Autodesk Inventor part; units mm, degrees
ref_plane "YZ Plane" through (0, 0, 0) normal (1, 0, 0) x (0, 1, 0)
ref_plane "XZ Plane" through (0, 0, 0) normal (0, 1, 0) x (-1, 0, 0)
ref_plane "XY Plane" through (0, 0, 0) normal (0, 0, 1) x (1, 0, 0)
sketch "Sketch3" plane through (0, 0, 0) normal (0, 0, 1) x (1, 0, 0)
  circle A0 centre (0, 0) radius 10.4
  circle A1 centre (-7.9, 0) radius 0.975
  circle A2 centre (7.9, 0) radius 0.975
  circle A3 centre (-7.9, 0) radius 0.975
  circle A4 centre (7.9, 0) radius 0.975
  dimension "d0" = 20.8
extrude "Extrusion1" add sketch "Sketch3" along normal blind 2.4
sketch "Sketch4" plane through (0, 0, 0) normal (0, 0, -1) x (-1, 0, 0)
  circle A0 centre (0, 0) radius 4.35
  circle A1 centre (0, 0) radius 2.7
  dimension "d3" = 8.7
  dimension "d4" = 5.4
extrude "Extrusion2" add sketch "Sketch4" along normal blind 3 contours A0 | A1
sketch "Sketch5" plane through (0, 0, -3) normal (0, 0, -1) x (-1, 0, 0)
  circle A0 centre (0, 0) radius 2.75
  dimension "d7" = 5.5
extrude "Extrusion3" cut sketch "Sketch5" against normal blind 2.1
sketch "Sketch6" plane through (0, 0, 2.4) normal (0, 0, 1) x (1, 0, 0)
  circle A0 centre (0, 0) radius 2.85
  dimension "d10" = 5.7
extrude "Extrusion4" cut sketch "Sketch6" against normal blind 1
sketch "Sketch7" plane through (0, 0, 1.4) normal (0, 0, 1) x (1, 0, 0)
  circle A0 centre (0, 0) radius 4.35
  circle A1 centre (0, 0) radius 1.5
  dimension "d13" = 3
extrude "Extrusion5" cut sketch "Sketch7" against normal through all contours A1
properties part number "Circulo_Inferior"
The listing builds one solid part. Answer for the finished solid, in the listing's coordinates (mm). A direction names the side the tool comes from. Coordinates: 2 decimals unless noted, no trailing zeros. Order: outer loops, then holes, each group sorted by start corner. A loop starts at its lowest first (then second) coordinate and runs counter-clockwise, first axis right, second up. Notation, with made-up numbers: (46.25, 55) -> (102.25, 55) arc R18 ccw to (102.25, 89) -> close; hole circle Ø10 at (36.25, 55). An arc over 180 degrees is marked (long way). Answer in a Markdown table with one row per item. Add a question column.
Item 1: Find section B-B (x = 0). Write down the section's boundary in (y, z).
Item 2: Find section C-C (z = -0.3). Write down the section's boundary in (x, y), then the cut area to 3 significant figures.
Item 3: Find section A-A (y = 0). Write down the section's boundary in (x, z) (3 decimals), then the cut area to 3 significant figures.
Item 4: Find the intervals of material crossed by L1, parallel to Y at x = 0, z = 1.75; L2, parallel to Y at x = 0, z = -2.25; L3, parallel to Z at x = -6.5, y = -4.25, in increasing order. Write a range as from..to.
Item 5: Determine the mould class of faces 1 (the face through (1.2, -1.2, 1.4)), 2 (the face through (0.943, 4.247, -1.479)), 3 (the face through (2.2, -2.2, 2.4)) for opening direction X: +X half, -X half, draft (parallel to the pull), parting line (faces both ways), or undercut.
Item 6: Which of the six approach directions +Z, -Z, +X, -X, +Y, -Y give full straight-line access (tool end or side, diameter ignored) to faces 4 (the face through (4.5, 0.1, 0)), 5 (the face through (-2.262, -1.734, 1.907)), 6 (the face through (8.83, -0.29, 1.18))?
Item 7: Find section D-D (y = -4). Write down the section's boundary in (x, z), then the cut area to 3 significant figures.
Item 8: Each of these flat-tipped pins is pushed along its axis until it touches: P1, Ø6.5, axis at x = -0.5, y = -1, coming from the +Z side; P2, Ø1, axis at x = -3, z = -2, coming from the +Y side; P3, Ø5, axis at x = 0, y = 0, coming from the -Z side; P4, Ø3, axis at x = -1.5, z = -1, coming from the -Y side. Where does it stop, or does it pass through?
Result set:
| question | item | result |
|---|---|---|
| 1 | outline | (-10.4, 0) -> (-4.35, 0) -> (-4.35, -3) -> (-2.75, -3) -> (-2.75, -0.9) -> (-1.5, -0.9) -> (-1.5, 1.4) -> (-2.85, 1.4) -> (-2.85, 2.4) -> (-10.4, 2.4) -> close; (1.5, -0.9) -> (2.75, -0.9) -> (2.75, -3) -> (4.35, -3) -> (4.35, 0) -> (10.4, 0) -> (10.4, 2.4) -> (2.85, 2.4) -> (2.85, 1.4) -> (1.5, 1.4) -> close |
| 2 | outline | circle Ø8.7 at (0, 0); hole circle Ø3 at (0, 0) |
| 2 | area | 52.4 mm² |
| 3 | outline | (-10.4, 0) -> (-8.875, 0) -> (-8.875, 2.4) -> (-10.4, 2.4) -> close; (-6.925, 0) -> (-4.35, 0) -> (-4.35, -3) -> (-2.75, -3) -> (-2.75, -0.9) -> (-1.5, -0.9) -> (-1.5, 1.4) -> (-2.85, 1.4) -> (-2.85, 2.4) -> (-6.925, 2.4) -> close; (1.5, -0.9) -> (2.75, -0.9) -> (2.75, -3) -> (4.35, -3) -> (4.35, 0) -> (6.925, 0) -> (6.925, 2.4) -> (2.85, 2.4) -> (2.85, 1.4) -> (1.5, 1.4) -> close; (8.875, 0) -> (10.4, 0) -> (10.4, 2.4) -> (8.875, 2.4) -> close |
| 3 | area | 42.5 mm² |
| 4 | L1 | y = -10.4..-2.85, 2.85..10.4 |
| 4 | L2 | y = -4.35..-2.75, 2.75..4.35 |
| 4 | L3 | z = 0..2.4 |
| 5 | face 1 | undercut |
| 5 | face 2 | parting line |
| 5 | face 3 | draft |
| 6 | face 4 | -Z |
| 6 | face 5 | +Z |
| 6 | face 6 | +Z, -Z |
| 7 | outline | (-9.6, 0) -> (-1.71, 0) -> (-1.71, -3) -> (1.71, -3) -> (1.71, 0) -> (9.6, 0) -> (9.6, 2.4) -> (-9.6, 2.4) -> close |
| 7 | area | 56.3 mm² |
| 8 | P1 | stops at z = 2.4 |
| 8 | P2 | stops at y = 3.56 |
| 8 | P3 | stops at z = -0.9 |
| 8 | P4 | stops at y = -10.39 |
